from build123d import *

# Parameters (mm, degrees)
SKETCH1_W           = 18.415
SKETCH1_H           = 230.1875
BOSS_EXTRUDE1_DEPTH = 9.525
SKETCH2_W           = 5.08
SKETCH2_H           = 216.8525
CUT_EXTRUDE1_DEPTH  = 1.27
SKETCH3_W           = 5.842
SKETCH3_H           = 7.62
SKETCH3_W_2         = 3.81
SKETCH3_H_2         = 4.064
SKETCH3_W_3         = 1.27
BOSS_EXTRUDE2_DEPTH = 8.128
SKETCH4_R           = 0.8255
BOSS_EXTRUDE3_DEPTH = 0.508
SKETCH5_W           = 5.08
SKETCH5_H           = 13.716
BOSS_EXTRUDE4_DEPTH = 2.794


with BuildPart() as part:
    # Sketch1 → Boss-Extrude1 (new body)
    with BuildSketch(Plane(origin=(0, 0, 0), x_dir=(1, 0, 0), z_dir=(0, 1, 0))):
        Rectangle(SKETCH1_W, SKETCH1_H)
    extrude(amount=BOSS_EXTRUDE1_DEPTH)

    # Sketch2 → Cut-Extrude1 (cut)
    with BuildSketch(Plane(origin=(0, 9.525, 0), x_dir=(1, 0, 0), z_dir=(0, 1, 0))):
        with Locations((-0.3175, 2.2225)):
            Rectangle(SKETCH2_W, SKETCH2_H)
    extrude(amount=-CUT_EXTRUDE1_DEPTH, mode=Mode.SUBTRACT)

    # Sketch3 → Boss-Extrude2 (add)
    with BuildSketch(Plane(origin=(0, 9.525, 0), x_dir=(1, 0, 0), z_dir=(0, 1, 0))):
        with Locations((-12.1285, 97.82175)):
            Rectangle(SKETCH3_W, SKETCH3_H)
        with Locations((-11.1125, 2.76225)):
            Rectangle(SKETCH3_W_2, SKETCH3_H_2)
        with Locations((-12.1285, -82.58175)):
            Rectangle(SKETCH3_W, SKETCH3_H)
        with Locations((9.8425, 111.28375)):
            Rectangle(SKETCH3_W_3, SKETCH3_H)
        with Locations((9.8425, -111.28375)):
            Rectangle(SKETCH3_W_3, SKETCH3_H)
    extrude(amount=-BOSS_EXTRUDE2_DEPTH)

    # Sketch4 → Boss-Extrude3 (add)
    with BuildSketch(Plane(origin=(0, 9.525, 0), x_dir=(1, 0, 0), z_dir=(0, 1, 0))):
        with Locations((-8.382, 113.82375)):
            Circle(SKETCH4_R)
        with Locations((8.382, 113.82375)):
            Circle(SKETCH4_R)
        with Locations((8.382, -113.82375)):
            Circle(SKETCH4_R)
        with Locations((-8.382, -113.82375)):
            Circle(SKETCH4_R)
    extrude(amount=BOSS_EXTRUDE3_DEPTH)

    # Sketch5 → Boss-Extrude4 (add)
    with BuildSketch(Plane.XZ):
        with Locations((4.3815, 94.11335)):
            Rectangle(SKETCH5_W, SKETCH5_H)
    extrude(amount=BOSS_EXTRUDE4_DEPTH)


solid = part.part
Input: part model. Units: mm. Frame: model coordinates. A direction names the side the tool comes from. Coordinates: 2 decimals unless noted, no trailing zeros. Loops run counter-clockwise (first coordinate to the right, second up) from the corner with the lowest first, then second, coordinate; pieces in that order, holes last.
(1) Pull-direction query (Z, two-part tool) for faces 5 (the face through (-9.208, 5, 2)), 6 (the face through (0, 5, 115.094)), 7 (the face through (-12, 1.397, -98)), 8 (the face through (3, 9.525, -2)); classes: released by +Z, released by -Z, zero draft, split by the parting line, or undercut.
(2) Section C-C on y = 3.75. Return the cut outline in (x, z).
(3) Section A-A on x = -1. Return the cut outline in (y, z) (3 decimals), then the cut area to 3 significant figures.
(4) Section B-B on z = -71.5. Return the cut outline in (x, y) (1 decimal).
(5) Set-up query: faces 1 (the face through (-12, 6, 86.392)), 2 (the face through (-12, 1.397, 83)), 3 (the face through (-12, 6, -94.012)), 4 (the face through (0, 8.255, -4)). Return all of +Z, -Z, +X, -X, +Y, -Y with unobstructed straight access to the full face (end or side cutting, diameter ignored); none if empty.
(6) Material intervals for probe 1 along Z at (x, y) = (-11, 7.25); probe 2 along X at (y, z) = (8.5, 0); probe 3 along X at (y, z) = (6.25, -77), sorted ascending.
(7) First-contact query: pin 1 Ø5 at (y, z) = (5, 23) entering from -X; pin 2 Ø3 at (x, z) = (-11, -96.5) entering from -Y; pin 3 Ø6 at (x, z) = (-12, 15) entering from -Y. Flat tips, straight axial feed; report the tip coordinate or a pass-through.
Data:
1. face 5: undercut
1. face 6: released by +Z
1. face 7: zero draft
1. face 8: undercut
2. outline: (-15.05, -101.63) - (-9.21, -101.63) - (-9.21, -115.09) - (10.48, -115.09) - (10.48, -107.47) - (9.21, -107.47) - (9.21, 107.47) - (10.48, 107.47) - (10.48, 115.09) - (-9.21, 115.09) - (-9.21, 86.39) - (-15.05, 86.39) - (-15.05, 78.77) - (-9.21, 78.77) - (-9.21, -0.73) - (-13.02, -0.73) - (-13.02, -4.79) - (-9.21, -4.79) - (-9.21, -94.01) - (-15.05, -94.01) - close
3. outline: (0, -115.094) - (9.525, -115.094) - (9.525, -110.649) - (8.255, -110.649) - (8.255, 106.204) - (9.525, 106.204) - (9.525, 115.094) - (0, 115.094) - close
3. area: 1,920 mm2
4. outline: (-9.2, 0) - (9.2, 0) - (9.2, 9.5) - (2.2, 9.5) - (2.2, 8.3) - (-2.9, 8.3) - (-2.9, 9.5) - (-9.2, 9.5) - close
5. face 1: +Z, -X, +Y, -Y
5. face 2: +Z, -Z, -X, -Y
5. face 3: -X, +Y, -Y
5. face 4: +Y
6. probe 1: z = -101.63 to -94.01, -4.79 to -0.73, 78.77 to 86.39
6. probe 2: x = -9.21 to -2.86, 2.22 to 9.21
6. probe 3: x = -9.21 to 9.21
7. pin 1: stops at x = -9.21
7. pin 2: stops at y = 1.4
7. pin 3: stops at y = 0
